from build123d import *

# Parameters (mm, degrees)
SKETCH2_W                 = 50.8
SKETCH2_H                 = 50.8
BOSS_EXTRUDE1_DEPTH       = 9.525
F_6_32_TAPPED_HOLE1_D     = 2.7051
F_6_32_TAPPED_HOLE1_DEPTH = 9.398
F_6_32_TAPPED_HOLE1_TIP   = 0.81269403
F_6_32_TAPPED_HOLE2_D     = 2.7051
F_6_32_TAPPED_HOLE2_DEPTH = 9.398
F_6_32_TAPPED_HOLE2_TIP   = 0.81269403
SKETCH3_R                 = 2.54
CUT_EXTRUDE1_DEPTH        = 58.589283942


with BuildPart() as part:
    # Sketch2 → Boss-Extrude1 (new body)
    with BuildSketch(Plane(origin=(0, 0, 0), x_dir=(1, 0, 0), z_dir=(0, 1, 0))):
        Rectangle(SKETCH2_W, SKETCH2_H)
    extrude(amount=BOSS_EXTRUDE1_DEPTH)

    # #6-32 Tapped Hole1
    with Locations(Plane.XY.offset(25.4)):
        with Locations((-20.32, 4.7625), (20.32, 4.7625)):
            Hole(F_6_32_TAPPED_HOLE1_D / 2, depth=F_6_32_TAPPED_HOLE1_DEPTH)
            with Locations((0, 0, -(F_6_32_TAPPED_HOLE1_DEPTH + F_6_32_TAPPED_HOLE1_TIP / 2))):  # 118° drill point
                Cone(0, F_6_32_TAPPED_HOLE1_D / 2, F_6_32_TAPPED_HOLE1_TIP, mode=Mode.SUBTRACT)

    # #6-32 Tapped Hole2
    with Locations(Plane(origin=(0, 0, -25.4), x_dir=(-1, 0, 0), z_dir=(0, 0, -1))):
        with Locations((-20.32, 4.7625), (20.32, 4.7625)):
            Hole(F_6_32_TAPPED_HOLE2_D / 2, depth=F_6_32_TAPPED_HOLE2_DEPTH)
            with Locations((0, 0, -(F_6_32_TAPPED_HOLE2_DEPTH + F_6_32_TAPPED_HOLE2_TIP / 2))):  # 118° drill point
                Cone(0, F_6_32_TAPPED_HOLE2_D / 2, F_6_32_TAPPED_HOLE2_TIP, mode=Mode.SUBTRACT)

    # Sketch3 → Cut-Extrude1 (cut, through all)
    with BuildSketch(Plane.XY.offset(25.4)):
        with Locations((20.32, 4.7625)):
            Circle(SKETCH3_R)
        with Locations((-20.32, 4.7625)):
            Circle(SKETCH3_R)
    extrude(amount=-CUT_EXTRUDE1_DEPTH, mode=Mode.SUBTRACT)


solid = part.part
Model file for the job. Use its own axes, mm. Round coordinates to 2 decimals unless told otherwise and drop trailing zeros. Loops run counter-clockwise (first coordinate to the right, second up) from the corner with the lowest first, then second, coordinate; pieces in that order, holes last. Notation, with made-up numbers: (54.5, 27) - (83.5, 27) arc R19 ccw to (83.5, 32) - close; hole circle Ø5 at (65, 72.5). An arc over 180 degrees is marked (long way). Write each question's results on one line, items separated by ' | '.
(1) Wall check: L1, parallel to X at y = 4.5, z = 1; L2, parallel to X at y = 4.75, z = -19.5; L3, parallel to Y at x = -20.32, z = -15 (1 decimal). Give the ranges that are in metal, low to high.
Answer below:
L1: x = -25.4 to -22.85, -17.79 to 17.79, 22.85 to 25.4 | L2: x = -25.4 to -22.86, -17.78 to 17.78, 22.86 to 25.4 | L3: y = 0 to 2.2, 7.3 to 9.5
(2) Mould opens along X. For faces 1 (the flat face through (-25.4, 5, 0)), 2 (the flat face through (0, 0, 0)), 3 (the cylindrical face through (17.782, 4.874, 0.356)), 4 (the cylindrical face through (-17.974, 3.79, 0.356)) say: released by +X, released by -X, zero draft, split by the parting line, or undercut.
Answer below:
face 1: released by -X | face 2: zero draft | face 3: undercut | face 4: undercut
(3) Saw through at C-C, the plane z = 5.5. List the corners of the cut face in (x, y) (1 decimal), then the cut area to 3 significant figures.
Answer below:
outline: (-25.4, 0) - (25.4, 0) - (25.4, 9.5) - (-25.4, 9.5) - close; hole circle Ø5.1 at (-20.3, 4.8); hole circle Ø5.1 at (20.3, 4.8) | area: 443 mm^2
(4) Saw through at A-A, the plane x = 20.32. List the corners of the cut face in (y, z) (1 decimal), then the cut area to 3 significant figures.
Answer below:
outline: (0, -25.4) - (2.2, -25.4) - (2.2, 25.4) - (0, 25.4) - close; (7.3, -25.4) - (9.5, -25.4) - (9.5, 25.4) - (7.3, 25.4) - close | area: 226 mm^2
(5) Saw through at B-B, the plane y = 6.5. List the corners of the cut face in (x, z), then the cut area to 3 significant figures.
Answer below:
outline: (-25.4, -25.4) - (-22.17, -25.4) - (-22.17, 25.4) - (-25.4, 25.4) - close; (-18.47, -25.4) - (18.47, -25.4) - (18.47, 25.4) - (-18.47, 25.4) - close; (22.17, -25.4) - (25.4, -25.4) - (25.4, 25.4) - (22.17, 25.4) - close | area: 2,200 mm^2
(6) Saw through at D-D, the plane y = 3. List the corners of the cut face in (x, z), then the cut area to 3 significant figures.
Answer below:
outline: (-25.4, -25.4) - (-22.15, -25.4) - (-22.15, 25.4) - (-25.4, 25.4) - close; (-18.49, -25.4) - (18.49, -25.4) - (18.49, 25.4) - (-18.49, 25.4) - close; (22.15, -25.4) - (25.4, -25.4) - (25.4, 25.4) - (22.15, 25.4) - close | area: 2,210 mm^2
(7) Pin check, flat tip, straight feed: pin 1 (3 mm diameter, centred on x = 20.32, y = 4.76, fed in from +Z). Stop position of the tip, or through.
Answer below:
pin 1: passes through
